Answer from the drawing. Dimensions are ordinates in mm from the lowest x, y and z of the part. A direction names the side the tool comes from. Round coordinates to 2 decimals unless told otherwise and drop trailing zeros. Loops run counter-clockwise (first coordinate to the right, second up) from the corner with the lowest first, then second, coordinate; pieces in that order, holes last. Notation, with made-up numbers: M 73.5,46 L 105.5,46 A7 ccw 105.5,50 Z; hole C -16.5,62.5 d6. An arc over 180 degrees is marked long. One line per item, written item: value.
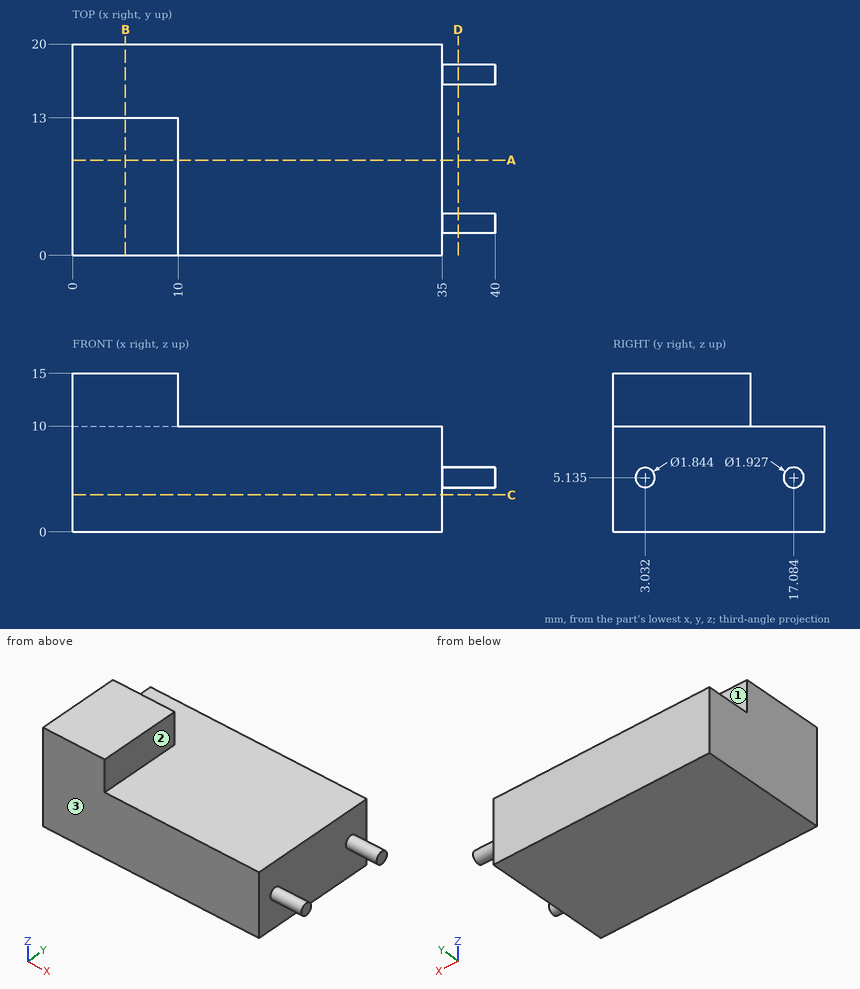
1) Find section A-A (y = 9). Give the vertices of the cut face in (x, z), then the cut area to 3 significant figures.
Check values:
outline: M 0,0 L 35,0 L 35,10 L 10,10 L 10,15 L 0,15 Z
area: 400 mm2
2) Each of these flat-tipped pins is pushed along its axis until it touches: pin 1 (5 mm diameter, centred on y = 6.5, z = 3, fed in from +X); pin 2 (1 mm diameter, centred on y = 14.5, z = 11.5, fed in from +X); pin 3 (1.5 mm diameter, centred on x = 28, y = 11.5, fed in from -Z); pin 4 (4 mm diameter, centred on x = 5, z = 13.5, fed in from +Y). Where does it stop, or does it pass through?
Check values:
pin 1: x = 35
pin 2: through
pin 3: z = 0
pin 4: y = 13
3) Find section D-D (x = 36.5). Give the vertices of the cut face in (y, z) (1 decimal).
Check values:
outline: C 3,5.1 d1.8; C 17.1,5.1 d1.9
4) Find section B-B (x = 5). Give the vertices of the cut face in (y, z).
Check values:
outline: M 0,0 L 20,0 L 20,10 L 13,10 L 13,15 L 0,15 Z
5) Find the intervals of material crossed by probe 1 along Z at (x, y) = (21.5, 17.5); probe 2 along X at (y, z) = (8, 7.5), in increasing order. Write a range as from..to.
Check values:
probe 1: 0..10
probe 2: 0..35
6) Find section C-C (z = 3.5). Give the vertices of the cut face in (x, y).
Check values:
outline: M 0,0 L 35,0 L 35,20 L 0,20 Z
7) For the marked faces 1, 2 and 3, determine the directions among +Z, -Z, +X, -X, +Y, -Y from which every point of the face is accessible in a straight line to the end or side of a thin tool.
Check values:
face 1: +Z, +X, -X, +Y
face 2: +Z, +X, +Y, -Y
face 3: +Z, -Z, +X, -X, -Y
